Verification items for the finished model (mm, model axes). A direction names the side the tool comes from. Give positions to 0.01 mm unless a question says otherwise; leave off trailing zeros. Order: outer loops, then holes, each group sorted by start corner. A loop starts at its lowest first (then second) coordinate and runs counter-clockwise, first axis right, second up. Notation, with made-up numbers: (12.25, 21.5) -> (29.25, 21.5) arc R28 cw to (29.25, 47.5) -> close; hole circle Ø9 at (5, 37.25). An arc over 180 degrees is marked (long way). Return JSON: item names as keys, results as strings. Group by question number.
(1) Cross-section at C-C on z = 123. Enter the section's corners in (x, y).
(2) Cross-section at A-A on x = 94.5. Enter the section's corners in (y, z), then the cut area to 4 significant figures.
(3) Cross-section at B-B on y = 58. Enter the section's corners in (x, z), then the cut area to 3 significant figures.
(4) Tool access check on faces 1 (the face through (-1, 62.5, -209)), 2 (the face through (102.5, 28, -209)), 3 (the face through (-102.5, 28, -209)). Record the directions out of +Z, -Z, +X, -X, +Y, -Y that give a thin tool (end or side, any length) a straight path to the whole face; none if there is none.
(5) Thickness scan on line 1 along Z through (x, y) = (3, 107.5); line 2 along Y through (x, z) = (3.5, 101.5); line 3 along Y through (x, z) = (-85, 103). Record the ranges inside material, lowest first.
(6) Depth check by flat-ended pin: pin 1 Ø1.5 at (x, z) = (-5, 84) entering from -Y; pin 2 Ø12 at (x, z) = (-102, -144.5) entering from -Y; pin 3 Ø3 at (x, z) = (21.5, -134) entering from -Y. Enter the tip coordinate at first touch or a pass-through.
(7) Cross-section at D-D on z = -135.5. Enter the section's corners in (x, y).
from build123d import *

# Parameters (mm, degrees)
F1_DEPTH = 130
F2_W     = 205
F2_H     = 90
F3_DEPTH = 80
F5_DEPTH = 232.501


with BuildPart() as f1:
    # F0 (on Right) → F1 (new body, symmetric)
    with BuildSketch(Plane.YZ):
        Polygon((117.5, 170), (-117.5, 170), (-42.5, -170), (117.5, -170), align=None)
    extrude(amount=F1_DEPTH, both=True)

    # F2 (on face) → F3 (join)
    with BuildSketch(Plane(origin=(0, 0, -170), x_dir=(1, 0, 0), z_dir=(0, 0, -1))):
        with Locations((0, -17.5)):
            Rectangle(F2_W, F2_H)
    extrude(amount=F3_DEPTH)

    # F4 (on face) → F5 (cut, through all)
    with BuildSketch(Plane(origin=(-102.5, 0, 0), x_dir=(0, -1, 0), z_dir=(-1, 0, 0))):
        Polygon((27.5, -250), (27.5, -170), (2.5, -250), align=None)
    extrude(amount=-F5_DEPTH, mode=Mode.SUBTRACT)


solid = f1.part
Verdict:
{
 "1": {"outline": "(-130, -107.13) -> (130, -107.13) -> (130, 117.5) -> (-130, 117.5) -> close"},
 "2": {"outline": "(-117.5, 170) -> (-42.5, -170) -> (-27.5, -170) -> (-2.5, -250) -> (62.5, -250) -> (62.5, -170) -> (117.5, -170) -> (117.5, 170) -> close", "area": "73,350 mm²"},
 "3": {"outline": "(-130, -170) -> (-102.5, -170) -> (-102.5, -250) -> (102.5, -250) -> (102.5, -170) -> (130, -170) -> (130, 170) -> (-130, 170) -> close", "area": "105,000 mm²"},
 "4": {"face 1": "-Z, +X, -X, +Y", "face 2": "-Z, +X, +Y, -Y", "face 3": "-Z, -X, +Y, -Y"},
 "5": {"line 1": "-170 to 170", "line 2": "-102.39 to 117.5", "line 3": "-102.72 to 117.5"},
 "6": {"pin 1": "y = -98.69", "pin 2": "y = -49.45", "pin 3": "y = -50.77"},
 "7": {"outline": "(-130, -50.11) -> (130, -50.11) -> (130, 117.5) -> (-130, 117.5) -> close"}
}
